Input: part model. Units: mm. Frame: model coordinates. A direction names the side the tool comes from. Round coordinates to 2 decimals unless told otherwise and drop trailing zeros. Loops run counter-clockwise (first coordinate to the right, second up) from the corner with the lowest first, then second, coordinate; pieces in that order, holes last.
(1) Cut plane A-A, the plane x = 0. Output: boundary loops of the cut face in (y, z), and give its area (3 significant figures).
(2) Line query: line 1 (Y direction, x = -5.25, z = -2.5); line 2 (X direction, y = 9.5, z = -8.5); line 3 (Z direction, x = -11, y = 1.5). Output: solid intervals per line, ascending.
(3) Cut plane B-B, the plane y = 19.5. Output: boundary loops of the cut face in (x, z), and give its area (3 significant figures).
(4) First-contact query: pin 1 Ø1 at (x, z) = (6, -2.5) entering from +Y; pin 2 Ø1.2 at (x, y) = (-11.5, 10) entering from -Z; pin 3 Ø4 at (y, z) = (12, 9) entering from -X. Flat tips, straight axial feed; report the tip coordinate or a pass-through.
(5) Cut plane D-D, the plane z = 11. Output: boundary loops of the cut face in (x, y), and give its area (3 significant figures).
(6) Access query for faces 1 (the face through (-11, 7, 12.376)), 2 (the face through (0, 12.656, 22)), 3 (the face through (10.02, 7, -1)). Directions: +Z, -Z, +X, -X, +Y, -Y. A direction counts if a zero-diameter tool reaches every point of the face in a straight line with its end or side. Return the directions, or none.
(7) Cut plane C-C, the plane z = 21.5. Output: boundary loops of the cut face in (x, y), and give its area (3 significant figures).
from build123d import *

# Parameters (mm, degrees)
SKETCH1_W           = 20.0406
SKETCH1_H           = 27.6987
SKETCH1_H_2         = 2.9464
SKETCH1_W_2         = 2.3495
BOSS_EXTRUDE1_DEPTH = 13.6779
SKETCH2_W           = 22.606
SKETCH2_H           = 11.6332
BOSS_EXTRUDE2_DEPTH = 13.4112
SKETCH3_R           = 1.4986
BOSS_EXTRUDE3_DEPTH = 9.906


with BuildPart() as part:
    # Sketch1 → Boss-Extrude1 (new body)
    with BuildSketch(Plane(origin=(0, 0, 0), x_dir=(1, 0, 0), z_dir=(0, 1, 0))):
        with Locations((0, 1.4732)):
            Rectangle(SKETCH1_W, SKETCH1_H)
        with Locations((0, -13.84935)):
            Rectangle(SKETCH1_W, SKETCH1_H_2)
        with Locations((-11.19505, -13.84935)):
            Rectangle(SKETCH1_W_2, SKETCH1_H_2)
        with Locations((11.19505, -13.84935)):
            Rectangle(SKETCH1_W_2, SKETCH1_H_2)
        with BuildLine():
            ThreePointArc((-10.0203, 15.32255), (0, 25.34285), (10.0203, 15.32255))
            Line((10.0203, 15.32255), (-10.0203, 15.32255))
        make_face()
    extrude(amount=BOSS_EXTRUDE1_DEPTH)

    # Sketch2 → Boss-Extrude2 (add)
    with BuildSketch(Plane.XY.offset(15.32255)):
        with Locations((0, 6.83895)):
            Rectangle(SKETCH2_W, SKETCH2_H)
    extrude(amount=BOSS_EXTRUDE2_DEPTH)

    # Sketch3 → Boss-Extrude3 (add)
    with BuildSketch(Plane(origin=(0, 13.6779, 0), x_dir=(1, 0, 0), z_dir=(0, 1, 0))):
        with Locations(Location((0, 15.32255, 0), (0, 0, 270))):
            Circle(SKETCH3_R)
    extrude(amount=BOSS_EXTRUDE3_DEPTH)


solid = part.part
Reported:
1. outline: (0, -25.34) - (13.68, -25.34) - (13.68, -16.82) - (23.58, -16.82) - (23.58, -13.82) - (13.68, -13.82) - (13.68, 15.32) - (12.66, 15.32) - (12.66, 28.73) - (1.02, 28.73) - (1.02, 15.32) - (0, 15.32) - close
1. area: 742 mm2
2. line 1: y = 0 to 13.68
2. line 2: x = -10.02 to 10.02
2. line 3: z = 12.38 to 28.73
3. outline: circle Ø3 at (0, -15.32)
3. area: 7.06 mm2
4. pin 1: stops at y = 13.68
4. pin 2: stops at z = 12.38
4. pin 3: stops at x = -10.02
5. outline: (-10.02, 0) - (10.02, 0) - (10.02, 13.68) - (-10.02, 13.68) - close
5. area: 274 mm2
6. face 1: -Z, -X, +Y, -Y
6. face 2: +Z, +X, -X, +Y
6. face 3: -Z, +X, +Y, -Y
7. outline: (-11.3, 1.02) - (11.3, 1.02) - (11.3, 12.66) - (-11.3, 12.66) - close
7. area: 263 mm2
